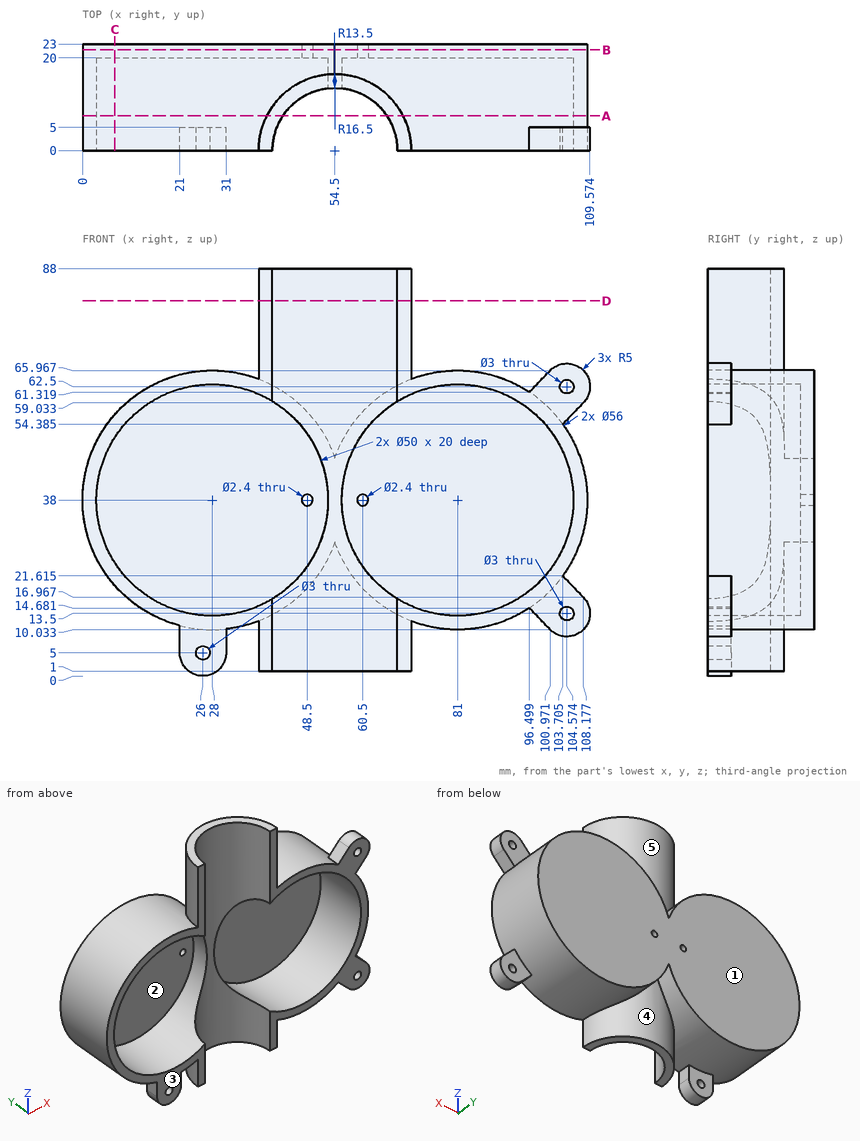
Source: three-view drawing plus pictorial views. Frame: mm from the lowest corner of the part. A direction names the side the tool comes from. Coordinates: 2 decimals unless noted, no trailing zeros. Order: outer loops, then holes, each group sorted by start corner. A loop starts at its lowest first (then second) coordinate and runs counter-clockwise, first axis right, second up. Notation, with made-up numbers: M 2.5,17 L 26.5,17 A16 cw 26.5,40 Z; hole C 53.25,-32.75 d1. An arc over 180 degrees is marked long. Write each question's results on one line, items separated by ' | '. Start each with the question number.
1. Pin query (flat end, axial travel): pin 1 (2.5 mm diameter, centred on x = 104.57, z = 62.5, fed in from -Y); pin 2 (1.5 mm diameter, centred on y = 3.5, z = 6.5, fed in from +X); pin 3 (3 mm diameter, centred on x = 60.5, z = 38, fed in from -Y); pin 4 (10 mm diameter, centred on x = 28, y = 15.5, fed in from +Z). Return the tip coordinate at first contact, or that it passes through.
2. Reachability of the marked faces 1, 2, 3, 4 and 5 from +Z, -Z, +X, -X, +Y, -Y: full face, straight path, thin tool, end or side. Return the list, or none.
3. Material intervals for L1, parallel to X at y = 22.2, z = 38; L2, parallel to Z at x = 81, y = 14.5; L3, parallel to Y at x = 89.5, z = 17, sorted ascending.
4. Section B-B, the plane y = 21.75. Return the cut outline in (x, z).
5. Section C-C, the plane x = 7. Return the cut outline in (y, z) (1 decimal), then the cut area to 3 significant figures.
6. Section A-A, the plane y = 7.5. Return the cut outline in (x, z) (1 decimal).
7. Section D-D, the plane z = 81. Return the cut outline in (x, y), then the cut area to 3 significant figures.
Solution:
1) pin 1: through | pin 2: x = 70.77 | pin 3: y = 20 | pin 4: z = 66
2) face 1: +Z, -Z, +X, -X, +Y | face 2: -Y | face 3: +Z, -Z, +X, -X, -Y | face 4: -Z, +Y | face 5: +Z, +Y
3) L1: 0 to 47.3, 49.7 to 59.3, 61.7 to 109 | L2: 10 to 13, 63 to 66 | L3: 20 to 23
4) outline: M 54.5,28.96 A28 ccw long 54.5,47.04 A28 ccw long Z; hole C 48.5,38 d2.4; hole C 60.5,38 d2.4
5) outline: M 0,19.5 L 23,19.5 L 23,56.5 L 0,56.5 L 0,51.6 L 20,51.6 L 20,24.4 L 0,24.4 Z | area: 309 mm²
6) outline: M 39.8,1 L 43.3,1 L 43.3,18.2 A25 cw long 43.3,57.8 L 43.3,88 L 39.8,88 L 39.8,63.4 A28 ccw long 39.8,12.6 Z; M 65.7,1 L 69.2,1 L 69.2,12.6 A28 ccw long 69.2,63.4 L 69.2,88 L 65.7,88 L 65.7,57.8 A25 cw long 65.7,18.2 Z
7) outline: M 38,0 L 41,0 A13.5 cw 68,0 L 71,0 A16.5 ccw Z | area: 141 mm²
